Input: part model. Units: mm. Frame: model coordinates. A direction names the side the tool comes from. Coordinates: 2 decimals unless noted, no trailing zeros. Order: outer loops, then holes, each group sorted by start corner. A loop starts at its lowest first (then second) coordinate and runs counter-clockwise, first axis right, second up. Notation, with made-up numbers: M 34,81 L 81,81 A34 cw 81,111 Z; hole C 62,17 d9. An arc over 180 degrees is marked long. Answer in a Markdown table with one row per item.
from build123d import *

# Parameters (mm, degrees)
SKETCH1_W           = 30
SKETCH1_H           = 30
BOSS_EXTRUDE1_DEPTH = 5
SKETCH2_R           = 11
CUT_EXTRUDE1_DEPTH  = 1
SKETCH5_W           = 30
SKETCH5_H           = 5
BOSS_EXTRUDE3_DEPTH = 33
SKETCH6_R           = 1.7
CUT_EXTRUDE2_DEPTH  = 9.378
SKETCH7_R           = 3
CUT_EXTRUDE3_DEPTH  = 9.378


with BuildPart() as part:
    # Sketch1 → Boss-Extrude1 (new body)
    with BuildSketch(Plane(origin=(0, 0, 0), x_dir=(1, 0, 0), z_dir=(0, 1, 0))):
        with Locations((0, -3.665024631)):
            Rectangle(SKETCH1_W, SKETCH1_H)
    extrude(amount=BOSS_EXTRUDE1_DEPTH)

    # Sketch2 → Cut-Extrude1 (cut)
    with BuildSketch(Plane(origin=(0, 5, 0), x_dir=(1, 0, 0), z_dir=(0, 1, 0))):
        with Locations(Location((0, -3.665024631, 0), (0, 0, 270))):
            Circle(SKETCH2_R)
    extrude(amount=-CUT_EXTRUDE1_DEPTH, mode=Mode.SUBTRACT)

    # Sketch5 → Boss-Extrude3 (add)
    with BuildSketch(Plane(origin=(0, 0, 0), x_dir=(1, 0, 0), z_dir=(0, 1, 0))):
        with Locations((0, 13.834975369)):
            Rectangle(SKETCH5_W, SKETCH5_H)
    extrude(amount=BOSS_EXTRUDE3_DEPTH)

    # Sketch6 → Cut-Extrude2 (cut)
    with BuildSketch(Plane.XY.offset(-11.334975369)):
        with Locations((-7.464356525, 12.532459144)):
            Circle(SKETCH6_R)
        with Locations((7.464356525, 12.532459144)):
            Circle(SKETCH6_R)
        with Locations((7.464356525, 25.467540856)):
            Circle(SKETCH6_R)
        with Locations((-7.464356525, 25.467540856)):
            Circle(SKETCH6_R)
    extrude(amount=-CUT_EXTRUDE2_DEPTH, mode=Mode.SUBTRACT)

    # Sketch7 → Cut-Extrude3 (cut)
    with BuildSketch(Plane(origin=(0, 4, 0), x_dir=(1, 0, 0), z_dir=(0, 1, 0))):
        with Locations(Location((0, -3.665024631, 0), (0, 0, 270))):
            Circle(SKETCH7_R)
    extrude(amount=-CUT_EXTRUDE3_DEPTH, mode=Mode.SUBTRACT)


solid = part.part
1) Reachability of faces 4 (the face through (0, 19, -11.335)), 5 (the face through (0.132, 2.028, 0.668)), 6 (the face through (-10.74, 4.51, 1.28)) from +Z, -Z, +X, -X, +Y, -Y: full face, straight path, thin tool, end or side. Return the list, or none.
Resolved:
| item | result |
|---|---|
| face 4 | +Z, +X, -X, +Y |
| face 5 | +Y, -Y |
| face 6 | +Y |
2) Mould query, pull axis X, two halves, no side actions, for faces 1 (the face through (-5.894, 11.881, -13.8)), 2 (the face through (15, 4, -7)), 3 (the face through (0, 33, -14)). Classes: +X half, -X half, draft (parallel to the pull), parting line (faces both ways), or undercut.
Resolved:
| item | result |
|---|---|
| face 1 | undercut |
| face 2 | +X half |
| face 3 | draft |
3) Cut plane D-D, the plane y = 9.5. Output: boundary loops of the cut face in (x, z).
Resolved:
| item | result |
|---|---|
| outline | M -15,-16.33 L 15,-16.33 L 15,-11.33 L -15,-11.33 Z |
4) Cut plane C-C, the plane z = -3. Output: boundary loops of the cut face in (x, y).
Resolved:
| item | result |
|---|---|
| outline | M -15,0 L 15,0 L 15,5 L 8.75,5 L 8.75,4 L -8.75,4 L -8.75,5 L -15,5 Z |
5) Contact query for flat-ended pins moving along their axis: pin 1 (8 mm diameter, centred on y = 26, z = -5, fed in from +X); pin 2 (17.5 mm diameter, centred on x = 0, z = 3.67, fed in from +Y); pin 3 (5.5 mm diameter, centred on x = 7.46, y = 25.47, fed in from +Z) (3 decimals); pin 4 (15 mm diameter, centred on x = -2.5, z = 9.5, fed in from +Y). Output: stop coordinate, or through.
Resolved:
| item | result |
|---|---|
| pin 1 | passes through |
| pin 2 | stops at y = 4 |
| pin 3 | stops at z = -11.335 |
| pin 4 | stops at y = 5 |
6) Cut plane B-B, the plane x = 7.75. Output: boundary loops of the cut face in (y, z), and give its area (3 significant figures).
Resolved:
| item | result |
|---|---|
| outline | M 0,-16.33 L 10.86,-16.33 L 10.86,-11.33 L 5,-11.33 L 5,-4.14 L 4,-4.14 L 4,11.47 L 5,11.47 L 5,18.67 L 0,18.67 Z; M 14.21,-16.33 L 23.79,-16.33 L 23.79,-11.33 L 14.21,-11.33 Z; M 27.14,-16.33 L 33,-16.33 L 33,-11.33 L 27.14,-11.33 Z |
| area | 266 mm2 |
7) Cut plane A-A, the plane x = 0. Output: boundary loops of the cut face in (y, z), and give its area (3 significant figures).
Resolved:
| item | result |
|---|---|
| outline | M 0,-16.33 L 33,-16.33 L 33,-11.33 L 5,-11.33 L 5,-7.33 L 4,-7.33 L 4,0.67 L 0,0.67 Z; M 0,6.67 L 4,6.67 L 4,14.67 L 5,14.67 L 5,18.67 L 0,18.67 Z |
| area | 269 mm2 |
8) Material intervals for probe 1 along Y at (x, z) = (-1.75, -6.5); probe 2 along Y at (x, z) = (10, -11); probe 3 along Z at (x, y) = (13, 28), sorted ascending.
Resolved:
| item | result |
|---|---|
| probe 1 | y = 0 to 4 |
| probe 2 | y = 0 to 5 |
| probe 3 | z = -16.33 to -11.33 |
